Autodesk Inventor part; units mm, degrees
ref_plane "YZ Plane" through (0, 0, 0) normal (1, 0, 0) x (0, 1, 0)
ref_plane "XZ Plane" through (0, 0, 0) normal (0, 1, 0) x (-1, 0, 0)
ref_plane "XY Plane" through (0, 0, 0) normal (0, 0, 1) x (1, 0, 0)
sketch "Sketch3" plane through (0, 0, 0) normal (0, 0, 1) x (1, 0, 0)
  circle A0 centre (0, 0) radius 22.5
  line L0 (-8.5, 0) -> (8.5, 0)
  line L1 (8.5, 0) -> (8.5, 75.5)
  line L2 (8.5, 75.5) -> (-8.5, 75.5)
  line L3 (-8.5, 75.5) -> (-8.5, 0)
  dimension "d5" = 45
  dimension "d6" = 75.5
  dimension "d7" = 17
extrude "Extrusion3" add sketch "Sketch3" along normal blind 15
sketch "Sketch4" plane through (0, 0, 0) normal (0, 0, -1) x (-1, 0, 0)
  arc A0 (-8.5, 20.8327) -> (8.5, 20.8327) centre (0, 0) ccw
  line L0 (8.5, 75.5) -> (8.5, 20.8327)
  line L1 (-8.5, 75.5) -> (8.5, 75.5)
  line L2 (-8.5, 20.8327) -> (-8.5, 75.5)
  arc A1 (-6.5, 19.4422) -> (6.5, 19.4422) centre (0, 0) ccw
  line L3 (-6.5, 19.4422) -> (-6.5, 73.5)
  line L4 (-6.5, 73.5) -> (6.5, 73.5)
  line L5 (6.5, 73.5) -> (6.5, 19.4422)
  dimension "d10" = 2
extrude "Extrusion4" cut sketch "Sketch4" against normal blind 13 contours L3 L4 L5 A1
chamfer "Chamfer1" distance 5 angle 45 1 edges at (0, 75.5, 15)
sketch "Sketch6" plane through (-8.5, 70.5, 15) normal (0, 0.7071068, 0.7071068) x (1, 0, 0)
  line L0 (2, 2.8284) -> (2, 4.2426)
  line L1 (2, 4.2426) -> (15, 4.2426)
  line L2 (15, 4.2426) -> (15, 2.8284)
  line L3 (15, 2.8284) -> (2, 2.8284)
  line L4 (0, 7.0711) -> (0, 0)
  line L5 (0, 0) -> (17, 0)
  line L6 (17, 0) -> (17, 7.0711)
  line L7 (17, 7.0711) -> (0, 7.0711)
  point P0 (8.5, -39.2444)
extrude "Extrusion5" add sketch "Sketch6" against normal blind 2 contours L0 L1 L2 L3 | L7 L6 L5 L4
properties part number "TARM10" material "ABS Plastic"
CAD build for the part. Positions are in the model's coordinates, mm. A direction names the side the tool comes from. Give positions to 0.01 mm unless a question says otherwise; leave off trailing zeros. Loops run counter-clockwise (first coordinate to the right, second up) from the corner with the lowest first, then second, coordinate; pieces in that order, holes last. Notation, with made-up numbers: (42.5, 1) - (72.5, 1) arc R14 ccw to (72.5, 13) - close; hole circle Ø11 at (14.25, 14.25). An arc over 180 degrees is marked (long way). Put each result on its own line as item: value.
Q1. Slice it at C-C (x = 0). Give the cut face in (y, z), plus the area to 3 significant figures.
Filled in:
outline: (-22.5, 0) - (-20.5, 0) - (-20.5, 13) - (69.67, 13) - (73.5, 9.17) - (73.5, 0) - (75.5, 0) - (75.5, 10) - (70.5, 15) - (-22.5, 15) - close
area: 243 mm²
Q2. Slice it at D-D (y = 0). Give the cut face in (x, z).
Filled in:
outline: (-22.5, 0) - (-20.5, 0) - (-20.5, 13) - (20.5, 13) - (20.5, 0) - (22.5, 0) - (22.5, 15) - (-22.5, 15) - close
Q3. Slice it at A-A (z = 3.25). Give the cut face in (x, y).
Filled in:
outline: (-8.5, 20.83) arc R22.5 ccw (long way) to (8.5, 20.83) - (8.5, 75.5) - (-8.5, 75.5) - close; hole (-6.5, 19.44) arc R20.5 ccw (long way) to (6.5, 19.44) - (6.5, 73.5) - (-6.5, 73.5) - close
Q4. Probe line 1 along X through (y, z) = (0, 10.75); line 2 along Y through (x, z) = (0, 7); line 3 along X through (y, z) = (64, 1.5). List the from-to ranges inside material, lowest first.
Filled in:
line 1: x = -22.5 to -20.5, 20.5 to 22.5
line 2: y = -22.5 to -20.5, 73.5 to 75.5
line 3: x = -8.5 to -6.5, 6.5 to 8.5
Q5. Flat gauge pins, fed straight in: pin 1 (1 mm diameter, centred on x = 13, z = 7, fed in from +Y); pin 2 (3 mm diameter, centred on y = 35.5, z = 8, fed in from +X); pin 3 (3 mm diameter, centred on y = 42, z = 3, fed in from -X). Where does each tip first touch, or does it go through?
Filled in:
pin 1: stops at y = 18.71
pin 2: stops at x = 8.5
pin 3: stops at x = -8.5
Q6. Tool access for faces 5 (the face through (6.5, 46, 6)), 6 (the face through (0.867, -22.483, 7.395)): list every direction of +Z, -Z, +X, -X, +Y, -Y with a clear straight run to the whole face (end or side of a thin tool).
Filled in:
face 5: -Z
face 6: +Z, -Z
Q7. Mould opens along X. For faces 1 (the face through (-8.5, 49, 7)), 2 (the face through (-6.5, 47, 6)), 3 (the face through (7, 30, 0)), 4 (the face through (8.5, 48, 7)) say: pulls with the +X half, pulls with the -X half, needs draft (parallel to the pull), parting line crosses it, or undercut.
Filled in:
face 1: pulls with the -X half
face 2: undercut
face 3: needs draft
face 4: pulls with the +X half
Q8. Slice it at B-B (y = 33.5). Give the cut face in (x, z), plus the area to 3 significant figures.
Filled in:
outline: (-8.5, 0) - (-6.5, 0) - (-6.5, 13) - (6.5, 13) - (6.5, 0) - (8.5, 0) - (8.5, 15) - (-8.5, 15) - close
area: 86.0 mm²
